The figure shows three views and two pictorial views of one solid part (mm, origin at its lowest corner). Answer the questions. A direction names the side the tool comes from. Coordinates: 2 decimals unless noted, no trailing zeros. Write each loop counter-clockwise with the first axis right and the second up, starting at its lowest first coordinate (ties: lowest second). Pieces come first, ordered by that corner, then holes.
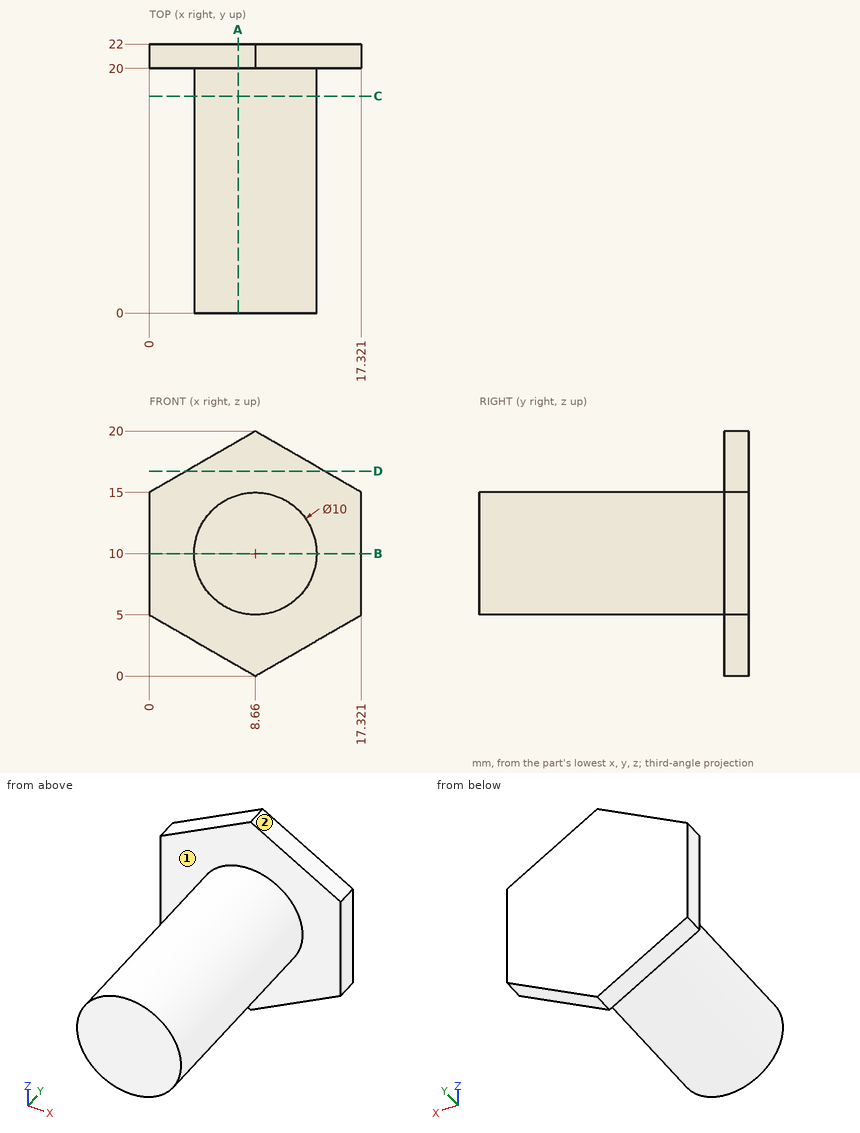
1. Section A-A on x = 7.25 is taken. Give the vertices of the cut face in (y, z) (1 decimal), then the cut area to 3 significant figures.
Results found:
outline: (0, 5.2) - (20, 5.2) - (20, 0.8) - (22, 0.8) - (22, 19.2) - (20, 19.2) - (20, 14.8) - (0, 14.8) - close
area: 229 mm2
2. Section C-C on y = 17.75 is taken. Give the vertices of the cut face in (x, z).
Results found:
outline: circle Ø10 at (8.66, 10)
3. Section B-B on z = 10 is taken. Give the vertices of the cut face in (x, y), then the cut area to 3 significant figures.
Results found:
outline: (0, 20) - (3.66, 20) - (3.66, 0) - (13.66, 0) - (13.66, 20) - (17.32, 20) - (17.32, 22) - (0, 22) - close
area: 235 mm2
4. A tool of negligible diameter and unlimited length cuts with its end or side. For the marked faces 1 and 2, from which of +Z, -Z, +X, -X, +Y, -Y can it reach the whole face along a straight path? Write none if from no direction.
Results found:
face 1: -Y
face 2: +Z, +X, +Y, -Y
5. Section D-D on z = 16.75 is taken. Give the vertices of the cut face in (x, y).
Results found:
outline: (3.03, 20) - (14.29, 20) - (14.29, 22) - (3.03, 22) - close
6. Find the intervals of material crossed by L1, parallel to Y at x = 15.5, z = 9.25; L2, parallel to X at y = 9, z = 10.25 (1 decimal); L3, parallel to Z at x = 8.75, y = 19.5, in increasing order.
Results found:
L1: y = 20 to 22
L2: x = 3.7 to 13.7
L3: z = 5 to 15
7. Flat-ended cylindrical pins translate along their axes: P1, Ø1.5, axis at x = 3.5, y = 5.5, coming from the -Z side (1 decimal); P2, Ø2, axis at x = 12, y = 17, coming from the -Z side; P3, Ø5, axis at y = 8, z = 14.5, coming from the -X side. Find the tip coordinate at first contact, or state that the pin passes through.
Results found:
P1: stops at z = 7.6
P2: stops at z = 5.58
P3: stops at x = 4.08
